```python
from build123d import *

# Parameters (mm, degrees)
F2_R     = 1
F3_SIZE  = 1
F5_DEPTH = 2.88


# Not quite as in the source:
# - a fillet or chamfer that OpenCascade refuses, or shapes differently, is made with other operations: its cross-section is extruded or revolved along the edge and cut away or added


with BuildPart() as f1:
    # F0 (on Front) → F1 (revolve)
    with BuildSketch(Plane.XZ):
        Polygon((-4, 0), (0, 0), (0, 21.056624327), (-2.5, 22.5), (-2.5, 28), (-6.5, 28), (-6.5, 20), (-4, 20), (-4, 16.25), (-3.5, 16), (-4, 15.75), align=None)
    revolve(axis=Axis((0, 0, 18.332445994), (0, 0, 1)))

    # F2
    f2_edges = [f1.edges().sort_by_distance(p)[0] for p in [
        (6.5, 0, 28),
    ]]
    fillet(f2_edges, radius=F2_R)

    # F3
    f3_edges = [f1.edges().sort_by_distance(p)[0] for p in [
        (4, 0, 0),
    ]]
    chamfer(f3_edges, length=F3_SIZE)

    # F4 (on face) → F5 (cut)
    with BuildSketch(Plane.XY.offset(28)):
        Polygon((-1.7320508076, -3), (1.7320508076, -3), (3.4641016151, 0), (1.7320508076, 3), (-1.7320508076, 3), (-3.4641016151, 0), align=None)
    extrude(amount=-F5_DEPTH, mode=Mode.SUBTRACT)

    # F6: chamfer of 1.5 x 2.5980762114 on 1 edges, made by hand


with BuildPart() as f6_tool2:
    # F6_s3 → F6_t4 (revolve)
    with BuildSketch(Plane.XZ):
        Polygon((-5.0980762114, 25.12), (-2.5, 23.62), (-2.5, 25.12), align=None)
    revolve(axis=Axis((0, 0, 25.12), (0, 0, 1)))

    split(bisect_by=Plane(origin=(-2.5980762114, -1.5, 0), x_dir=(0, 0, 1), z_dir=(0.8660254038, 0.5, 0)), keep=Keep.TOP)

    split(bisect_by=Plane(origin=(-2.5980762114, 1.5, 0), x_dir=(0, 0, 1), z_dir=(0.8660254038, -0.5, 0)), keep=Keep.TOP)

    split(bisect_by=Plane.XZ.offset(-3), keep=Keep.TOP)

    split(bisect_by=Plane(origin=(2.5980762114, 1.5, 0), x_dir=(0, 0, 1), z_dir=(-0.8660254038, -0.5, 0)), keep=Keep.TOP)

    split(bisect_by=Plane(origin=(2.5980762114, -1.5, 0), x_dir=(0, 0, 1), z_dir=(-0.8660254038, 0.5, 0)), keep=Keep.TOP)

    split(bisect_by=Plane.XZ.offset(3), keep=Keep.BOTTOM)


with BuildPart() as f1_1:
    add(f1.part)

    # F6_t1: cut F6_tool2
    add(f6_tool2.part, mode=Mode.SUBTRACT)


solid = f1_1.part
```
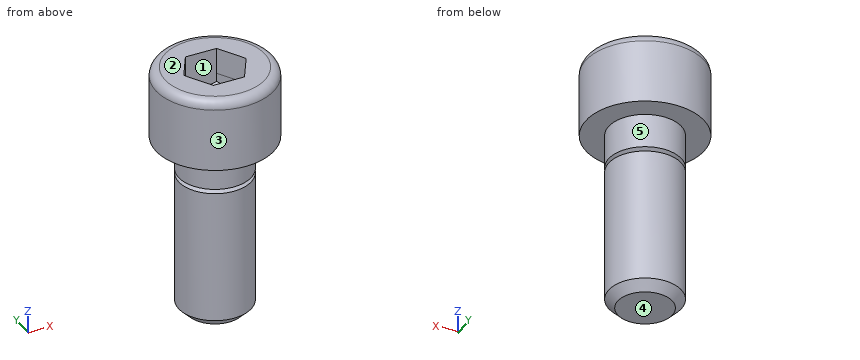
Here's how the part is built. I have some questions about the finished solid (model axes, mm). Face numbers are marked on the shaded views. A direction names the side the tool comes from. Give positions to 0.01 mm unless a question says otherwise; leave off trailing zeros. Use one line per item in the form item = value. Start each with the question number.
Q1. Which directions (+Z, -Z, +X, -X, +Y, -Y) give clear straight access to the entire face, cutting with the end or side of a thin tool? Please do the marked faces 4 and 5.
Q2. I need wall thicknesses on line 1 along Y through (x, z) = (0, 22.8); line 2 along Y through (x, z) = (5.5, 22.75). Which ranges of each line are inside material? Lowest first, please.
Q3. Thinking about a two-plate mould opening in Y: for the marked faces 1, 2 and 3, which applies, +Y half, -Y half, draft (parallel to the pull), parting line (faces both ways), or undercut?
Q4. Will these pins go through, and if not, where does the flat tip stop? pin 1 Ø1 at (x, y) = (-4.5, 3) entering from -Z; pin 2 Ø2 at (y, z) = (3, 15.5) entering from -X; pin 3 Ø3 at (y, z) = (-1.5, 18) entering from +X.
Taken from the geometry:
q1.face_4 = -Z, +X, -X, +Y, -Y
q1.face_5 = -Z
q2.line_1 = -6.5 to -2.5, 2.5 to 6.5
q2.line_2 = -3.46 to 3.46
q3.face_1 = undercut
q3.face_2 = draft
q3.face_3 = parting line
q4.pin_1 = 20
q4.pin_2 = -3.46
q4.pin_3 = 4
